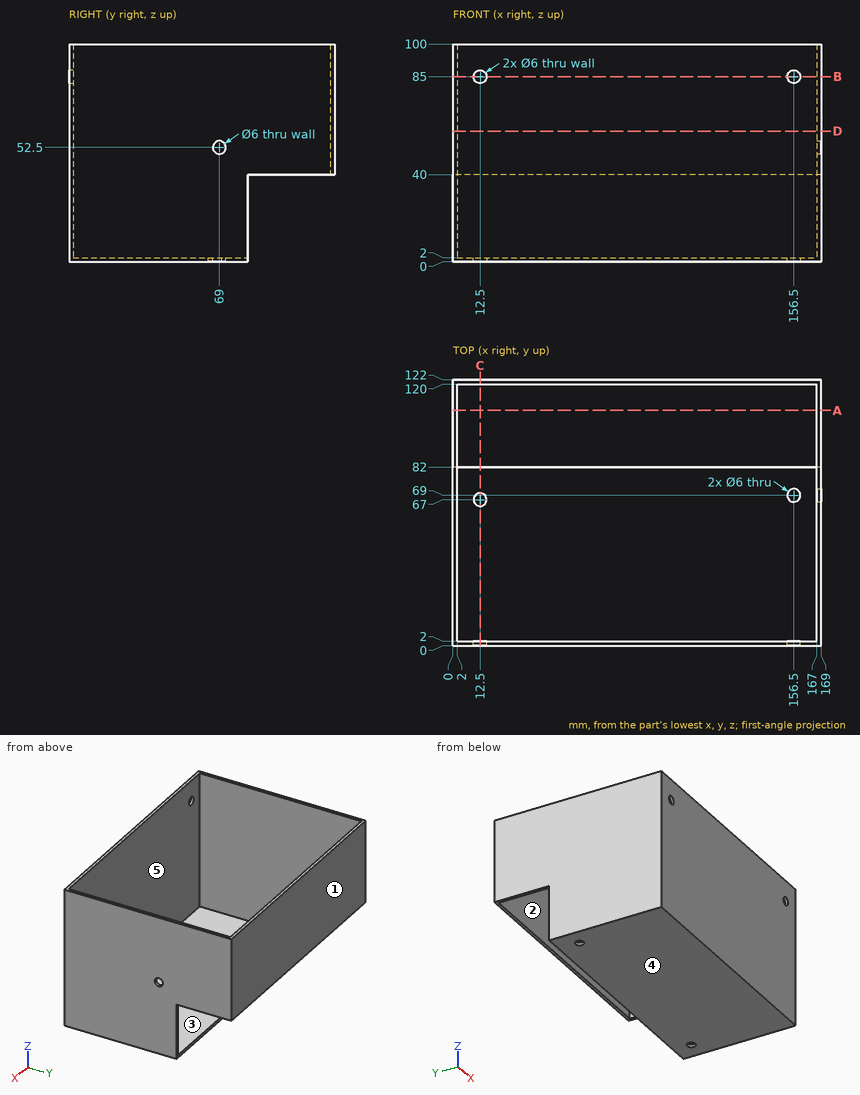
Verification items for this drawing (mm, ordinates from the low corner). A direction names the side the tool comes from. Coordinates: 2 decimals unless noted, no trailing zeros. Order: outer loops, then holes, each group sorted by start corner. A loop starts at its lowest first (then second) coordinate and runs counter-clockwise, first axis right, second up. Notation, with made-up numbers: (88.5, 22.5) - (92.5, 22.5) arc R28 ccw to (92.5, 58.5) - close; hole circle Ø3 at (-9, -15). An arc over 180 degrees is marked (long way). Answer in a Markdown table with one row per item. Add a question column.
1. Draft check along Y on the marked faces 1, 2 and 3. Enter one of: +Y half, -Y half, draft (parallel to the pull), parting line (faces both ways), or undercut.
2. Section check A-A (y = 108). Enter the section's corners in (x, z).
3. Gauge pin test, flat ends, axial feed: pin 1 Ø1 at (x, y) = (37, 16) entering from +Z; pin 2 Ø5 at (x, z) = (40.5, 36.5) entering from +Y; pin 3 Ø5 at (x, z) = (12.5, 85) entering from -Y. Record the tip position at first contact, or that the pin passes through.
4. Access from +Z, -Z, +X, -X, +Y, -Y to the whole of each face (thin tool, end or side, straight path). Record for the marked faces 4 and 5.
5. Section check B-B (z = 85). Enter the section's corners in (x, y).
6. Section check C-C (x = 12.5). Enter the section's corners in (y, z).
7. Material ranges on L1, parallel to X at y = 1.3, z = 85; L2, parallel to X at y = 105, z = 60.5; L3, parallel to Y at x = 132, z = 92.5, recorded low to high. Write a range as [from, to].
8. Section check D-D (z = 60). Enter the section's corners in (x, y), plus the area to 3 significant figures.
Data:
| question | item | result |
|---|---|---|
| 1 | face 1 | +Y half |
| 1 | face 2 | undercut |
| 1 | face 3 | draft |
| 2 | outline | (0, 40) - (2, 40) - (2, 100) - (0, 100) - close; (167, 40) - (169, 40) - (169, 100) - (167, 100) - close |
| 3 | pin 1 | stops at z = 2 |
| 3 | pin 2 | stops at y = 2 |
| 3 | pin 3 | stops at y = 120 |
| 4 | face 4 | -Z, +X, -X, +Y, -Y |
| 4 | face 5 | +Z |
| 5 | outline | (0, 0) - (9.5, 0) - (9.5, 2) - (2, 2) - (2, 120) - (167, 120) - (167, 2) - (159.5, 2) - (159.5, 0) - (169, 0) - (169, 122) - (0, 122) - close; (15.5, 0) - (153.5, 0) - (153.5, 2) - (15.5, 2) - close |
| 6 | outline | (0, 0) - (64, 0) - (64, 2) - (2, 2) - (2, 82) - (0, 82) - close; (0, 88) - (2, 88) - (2, 100) - (0, 100) - close; (70, 0) - (82, 0) - (82, 2) - (70, 2) - close; (120, 40) - (122, 40) - (122, 100) - (120, 100) - close |
| 7 | L1 | x = [0, 9.5], [15.5, 153.5], [159.5, 169] |
| 7 | L2 | x = [0, 2], [167, 169] |
| 7 | L3 | y = [0, 2], [120, 122] |
| 8 | outline | (0, 0) - (169, 0) - (169, 122) - (0, 122) - close; hole (2, 2) - (167, 2) - (167, 120) - (2, 120) - close |
| 8 | area | 1,150 mm² |
